```python
from build123d import *

# Parameters (mm, degrees)
S01_BEARING_BARREL_R                             = 22
F_01_BEARING_BARREL_DEPTH                        = 21
F_02_TORQUE_ARM_1_DEPTH                          = 10
F_03_TORQUE_ARM_2_DEPTH                          = 10
F_04_TORQUE_ARM_3_DEPTH                          = 10
F_05_WHEEL_ARM_ROOT_TO_ROUNDED_ELBOW_DEPTH       = 10
F_06_LONG_DROPPED_WHEEL_ARM_DEPTH                = 10
F_07_BROAD_CAM_FOLLOWER_MOUNTING_LUG_DEPTH       = 10
F_08_START                                       = -1
S08_BEARING_THROUGH_RELIEF_R                     = 12
F_08_BEARING_THROUGH_RELIEF_DEPTH                = 23
F_09_START                                       = -0.1
S09_INBOARD_6001_SEAT_R                          = 14.1
F_09_INBOARD_6001_SEAT_DEPTH                     = 8.2
F_10_START                                       = 12.9
S10_OUTBOARD_6001_SEAT_R                         = 14.1
F_10_OUTBOARD_6001_SEAT_DEPTH                    = 8.2
F_11_START                                       = -1
S11_KEEPER_SCREWS_R                              = 1.7
F_11_KEEPER_SCREWS_DEPTH                         = 23
F_12_START                                       = -1
S12_TORQUE_PIN_RETAINING_STEMS_R                 = 3.25
F_12_TORQUE_PIN_RETAINING_STEMS_DEPTH            = 12
F_19_START                                       = -1
S19_THROUGH_BORE_FOR_STEEL_FOLLOWER_BU_R         = 5.1
F_19_THROUGH_BORE_FOR_STEEL_FOLLOWER_BUS_DEPTH   = 12
F_20_START                                       = -0.1
S20_FLUSH_SEAT_FOR_BUSH_FLANGE_R                 = 7.6
F_20_FLUSH_SEAT_FOR_BUSH_FLANGE_DEPTH            = 2.1
FLAT_MOTOR_MOUNTING_PAD_LAYOUT_R                 = 21
FLAT_MOTOR_MOUNTING_PAD_DEPTH                    = 10
R4_BLENDS_FROM_ARM_INTO_MOTOR_PAD_R              = 4
F_28_START                                       = 10.12
F_28_X_14_CLOSED_THROUGH_SLOT_FOR_MOTOR_OU_DEPTH = 10.24
SIX_START                                        = 10.12
SIX_CLEARANCE_HOLES_FROM_JOHNSON_MOT_2_R         = 1.65
SIX_CLEARANCE_HOLES_FROM_JOHNSON_MOTOR_F_DEPTH   = 10.24


with BuildPart() as part:
    # S01 - Bearing barrel → 01 - Bearing barrel (new body)
    with BuildSketch(Plane.XY):
        with Locations(Location((0, 0, 0), (0, 0, 180))):
            Circle(S01_BEARING_BARREL_R)
    extrude(amount=F_01_BEARING_BARREL_DEPTH)

    # S02 - Torque arm 1 → 02 - Torque arm 1 (add)
    with BuildSketch(Plane.XY):
        with BuildLine():
            Line((0, 8), (36, 8))
            ThreePointArc((36, 8), (44, 0), (36, -8))
            Line((36, -8), (0, -8))
            ThreePointArc((0, -8), (-8, 0), (0, 8))
        make_face()
    extrude(amount=F_02_TORQUE_ARM_1_DEPTH)

    # S03 - Torque arm 2 → 03 - Torque arm 2 (add)
    with BuildSketch(Plane.XY):
        with BuildLine():
            Line((-6.92820323, -4), (-24.92820323, 27.176914536))
            ThreePointArc((-24.92820323, 27.176914536), (-22, 38.105117767), (-11.07179677, 35.176914536))
            Line((-11.07179677, 35.176914536), (6.92820323, 4))
            ThreePointArc((6.92820323, 4), (4, -6.92820323), (-6.92820323, -4))
        make_face()
    extrude(amount=F_03_TORQUE_ARM_2_DEPTH)

    # S04 - Torque arm 3 → 04 - Torque arm 3 (add)
    with BuildSketch(Plane.XY):
        with BuildLine():
            Line((6.92820323, -4), (-11.07179677, -35.176914536))
            ThreePointArc((-11.07179677, -35.176914536), (-22, -38.105117767), (-24.92820323, -27.176914536))
            Line((-24.92820323, -27.176914536), (-6.92820323, 4))
            ThreePointArc((-6.92820323, 4), (4, 6.92820323), (6.92820323, -4))
        make_face()
    extrude(amount=F_04_TORQUE_ARM_3_DEPTH)

    # S05 - Wheel arm root to rounded elbow → 05 - Wheel arm root to rounded elbow (add)
    with BuildSketch(Plane.XY):
        with BuildLine():
            Line((0.890943823, 12.969434032), (67.022341031, 8.426494092))
            ThreePointArc((67.022341031, 8.426494092), (79.10083124, -5.433883763), (65.240453385, -17.512373972))
            Line((65.240453385, -17.512373972), (-0.890943823, -12.969434032))
            ThreePointArc((-0.890943823, -12.969434032), (-12.969434032, 0.890943823), (0.890943823, 12.969434032))
        make_face()
    extrude(amount=F_05_WHEEL_ARM_ROOT_TO_ROUNDED_ELBOW_DEPTH)

    # S06 - Long dropped wheel arm → 06 - Long dropped wheel arm (add)
    with BuildSketch(Plane.XY):
        with BuildLine():
            Line((76.528125799, 1.449391376), (116.886494349, -68.572605409))
            ThreePointArc((116.886494349, -68.572605409), (112.482097074, -84.961665317), (96.093037167, -80.557268042))
            Line((96.093037167, -80.557268042), (55.734668617, -10.535271257))
            ThreePointArc((55.734668617, -10.535271257), (60.139065892, 5.853788651), (76.528125799, 1.449391376))
        make_face()
    extrude(amount=F_06_LONG_DROPPED_WHEEL_ARM_DEPTH)

    # S07 - Broad cam follower mounting lug → 07 - Broad cam follower mounting lug (add)
    with BuildSketch(Plane.XY):
        with BuildLine():
            Line((6.53566842, 10.064046815), (57.694573065, -23.158934321))
            ThreePointArc((57.694573065, -23.158934321), (61.22295146, -39.758649556), (44.623236224, -43.287027951))
            Line((44.623236224, -43.287027951), (-6.53566842, -10.064046815))
            ThreePointArc((-6.53566842, -10.064046815), (-10.064046815, 6.53566842), (6.53566842, 10.064046815))
        make_face()
    extrude(amount=F_07_BROAD_CAM_FOLLOWER_MOUNTING_LUG_DEPTH)

    # S08 - Bearing through relief → 08 - Bearing through relief (cut)
    with BuildSketch(Plane.XY.offset(F_08_START)):
        Circle(S08_BEARING_THROUGH_RELIEF_R)
    extrude(amount=F_08_BEARING_THROUGH_RELIEF_DEPTH, mode=Mode.SUBTRACT)

    # S09 - Inboard 6001 seat → 09 - Inboard 6001 seat (cut)
    with BuildSketch(Plane.XY.offset(F_09_START)):
        Circle(S09_INBOARD_6001_SEAT_R)
    extrude(amount=F_09_INBOARD_6001_SEAT_DEPTH, mode=Mode.SUBTRACT)

    # S10 - Outboard 6001 seat → 10 - Outboard 6001 seat (cut)
    with BuildSketch(Plane.XY.offset(F_10_START)):
        Circle(S10_OUTBOARD_6001_SEAT_R)
    extrude(amount=F_10_OUTBOARD_6001_SEAT_DEPTH, mode=Mode.SUBTRACT)

    # S11 - Keeper screws → 11 - Keeper screws (cut)
    with BuildSketch(Plane.XY.offset(F_11_START)):
        with Locations((0, 18.25)):
            Circle(S11_KEEPER_SCREWS_R)
        with Locations((-15.804963619, -9.125)):
            Circle(S11_KEEPER_SCREWS_R)
        with Locations((15.804963619, -9.125)):
            Circle(S11_KEEPER_SCREWS_R)
    extrude(amount=F_11_KEEPER_SCREWS_DEPTH, mode=Mode.SUBTRACT)

    # S12 - Torque pin retaining stems → 12 - Torque pin retaining stems (cut)
    with BuildSketch(Plane.XY.offset(F_12_START)):
        with Locations(Location((36, 0, 0), (0, 0, 180))):
            Circle(S12_TORQUE_PIN_RETAINING_STEMS_R)
        with Locations(Location((-18, 31.176914536, 0), (0, 0, 180))):
            Circle(S12_TORQUE_PIN_RETAINING_STEMS_R)
        with Locations(Location((-18, -31.176914536, 0), (0, 0, 180))):
            Circle(S12_TORQUE_PIN_RETAINING_STEMS_R)
    extrude(amount=F_12_TORQUE_PIN_RETAINING_STEMS_DEPTH, mode=Mode.SUBTRACT)

    # S19 - Through bore for steel follower bu → 19 - Through bore for steel follower bus (cut)
    with BuildSketch(Plane.XY.offset(F_19_START)):
        with Locations(Location((51.158904645, -33.222981136, 0), (0, 0, 180))):
            Circle(S19_THROUGH_BORE_FOR_STEEL_FOLLOWER_BU_R)
    extrude(amount=F_19_THROUGH_BORE_FOR_STEEL_FOLLOWER_BUS_DEPTH, mode=Mode.SUBTRACT)

    # S20 - Flush seat for bush flange → 20 - Flush seat for bush flange (cut)
    with BuildSketch(Plane.XY.offset(F_20_START)):
        with Locations((51.158904645, -33.222981136)):
            Circle(S20_FLUSH_SEAT_FOR_BUSH_FLANGE_R)
    extrude(amount=F_20_FLUSH_SEAT_FOR_BUSH_FLANGE_DEPTH, mode=Mode.SUBTRACT)

    # Flat motor mounting pad layout → Flat motor mounting pad (add)
    with BuildSketch(Plane.XY):
        with Locations((106.780015642, -75.748703358)):
            Circle(FLAT_MOTOR_MOUNTING_PAD_LAYOUT_R)
    extrude(amount=FLAT_MOTOR_MOUNTING_PAD_DEPTH)

    # R4 blends from arm into motor pad
    r4_blends_from_arm_into_motor_pad_edges = [part.edges().sort_by_distance(p)[0] for p in [
        (108.985808176, -54.864870393, 5),
        (87.956079001, -66.439599786, 5),
    ]]
    fillet(r4_blends_from_arm_into_motor_pad_edges, radius=R4_BLENDS_FROM_ARM_INTO_MOTOR_PAD_R)

    # Original round-ended output slot layout → 28 x 14 closed through slot for motor ou (cut)
    with BuildSketch(Plane.XY.offset(F_28_START)):
        with BuildLine():
            Line((96.668388671, -75.960835392), (106.567883608, -66.061340455))
            ThreePointArc((106.567883608, -66.061340455), (116.467378544, -66.061340455), (116.467378544, -75.960835392))
            Line((116.467378544, -75.960835392), (106.567883608, -85.860330328))
            ThreePointArc((106.567883608, -85.860330328), (96.668388671, -85.860330328), (96.668388671, -75.960835392))
        make_face()
    extrude(amount=-F_28_X_14_CLOSED_THROUGH_SLOT_FOR_MOTOR_OU_DEPTH, mode=Mode.SUBTRACT)

    # Six clearance holes from Johnson mot 2 → Six clearance holes from Johnson motor f (cut)
    with BuildSketch(Plane.XY.offset(SIX_START)):
        with Locations((92.035157904, -79.699576081)):
            Circle(SIX_CLEARANCE_HOLES_FROM_JOHNSON_MOT_2_R)
        with Locations((102.829142919, -90.493561096)):
            Circle(SIX_CLEARANCE_HOLES_FROM_JOHNSON_MOT_2_R)
        with Locations((117.574000657, -86.542688372)):
            Circle(SIX_CLEARANCE_HOLES_FROM_JOHNSON_MOT_2_R)
        with Locations((121.52487338, -71.797830634)):
            Circle(SIX_CLEARANCE_HOLES_FROM_JOHNSON_MOT_2_R)
        with Locations((110.730888366, -61.003845619)):
            Circle(SIX_CLEARANCE_HOLES_FROM_JOHNSON_MOT_2_R)
        with Locations((95.986030627, -64.954718343)):
            Circle(SIX_CLEARANCE_HOLES_FROM_JOHNSON_MOT_2_R)
    extrude(amount=-SIX_CLEARANCE_HOLES_FROM_JOHNSON_MOTOR_F_DEPTH, mode=Mode.SUBTRACT)


solid = part.part
```
Can you work these out from the model? Positions are in its coordinate system, mm. A direction names the side the tool comes from. Coordinates: 2 decimals unless noted, no trailing zeros. Loops run counter-clockwise (first coordinate to the right, second up) from the corner with the lowest first, then second, coordinate; pieces in that order, holes last.
1) I need wall thicknesses on probe 1 along Y at (x, z) = (49, 5.5); probe 2 along X at (y, z) = (-9, 11); probe 3 along Y at (x, z) = (47.5, 2.5). Which ranges of each line are inside material? Lowest first, please.
2) Which directions (+Z, -Z, +X, -X, +Y, -Y) give clear straight access to the entire face, cutting with the end or side of a thin tool? Please do faces 1 (the cylindrical face through (6.506, -12.509, 3.993)), 2 (the flat face through (-7.14, -28.37, 4.93)), 3 (the cylindrical face through (6.506, -12.509, 16.893)).
3) For pin 1 (2 mm diameter, centred on x = -8.5, z = 8.5, fed in from -Y); pin 2 (18 mm diameter, centred on x = -15.5, y = -31.5, fed in from +Z); pin 3 (1.5 mm diameter, centred on y = -38, z = 8, fed in from +X), each with a flat end and sliding along its axis, tell me the tip position at first contact or that it passes through.
4) Thinking about a two-plate mould opening in Y: for faces 4 (the cylindrical face through (-17.58, -34.4, 4.93)), 5 (the flat face through (27.03, -31.86, 4.93)), 6 (the flat face through (68, -30, 10)), which applies, pulls with the +Y half, pulls with the -Y half, needs draft (parallel to the pull), parting line crosses it, or undercut?
5) Imagine slicing it at C-C on y = 18.25. List the corners of the cut face in (x, z) for me.
6) Imagine slicing it at B-B on x = 36. List the corners of the cut face in (y, z) for me.
7) Imagine slicing it at D-D on z = 16.5. List the corners of the cut face in (x, y) for me (3 decimals), plus the area to 3 significant figures.
8) Imagine slicing it at A-A on x = 0. List the corners of the cut face in (y, z) for me, plus the area to 3 significant figures.
Completed:
1. probe 1: y = -45.03 to -37.84, -28.6 to -17.51, -16.4 to 9.66
1. probe 2: x = -20.07 to -17.5, -14.11 to -7.94, 7.94 to 14.11, 17.5 to 20.07
1. probe 3: y = -44.65 to -36.78, -29.67 to -16.54, -16.29 to 9.77
2. face 1: -Z
2. face 2: +Z, -Z, -Y
2. face 3: +Z
3. pin 1: stops at y = -32.45
3. pin 2: stops at z = 10
3. pin 3: stops at x = 99.7
4. face 4: undercut
4. face 5: pulls with the -Y half
4. face 6: needs draft
5. outline: (-19.77, 0) - (-1.7, 0) - (-1.7, 21) - (-12.29, 21) - (-12.29, 10) - (-19.77, 10) - close; (1.7, 0) - (12.29, 0) - (12.29, 21) - (1.7, 21) - close
6. outline: (-37.69, 0) - (-3.25, 0) - (-3.25, 10) - (-37.69, 10) - close; (3.25, 0) - (10.56, 0) - (10.56, 10) - (3.25, 10) - close
7. outline: circle Ø44 at (0, 0); hole circle Ø3.4 at (-15.805, -9.125); hole circle Ø28.2 at (0, 0); hole circle Ø3.4 at (0, 18.25); hole circle Ø3.4 at (15.805, -9.125)
7. area: 869 mm2
8. outline: (-22, 0) - (-14.1, 0) - (-14.1, 8.1) - (-12, 8.1) - (-12, 12.9) - (-14.1, 12.9) - (-14.1, 21) - (-22, 21) - close; (12, 8.1) - (14.1, 8.1) - (14.1, 0) - (16.55, 0) - (16.55, 21) - (14.1, 21) - (14.1, 12.9) - (12, 12.9) - close; (19.95, 0) - (22, 0) - (22, 21) - (19.95, 21) - close
8. area: 281 mm2
